Autodesk Inventor part; units mm, degrees
ref_plane "YZ Plane" through (0, 0, 0) normal (1, 0, 0) x (0, 1, 0)
ref_plane "XZ Plane" through (0, 0, 0) normal (0, 1, 0) x (-1, 0, 0)
ref_plane "XY Plane" through (0, 0, 0) normal (0, 0, 1) x (1, 0, 0)
sketch "Sketch1" plane through (0, 0, 0) normal (0, 1, 0) x (-1, 0, 0)
  circle A0 centre (0, 0) radius 20
  circle A1 centre (20, 0) radius 2
  circle A2 centre (10, 17.3205) radius 2
  circle A3 centre (-10, 17.3205) radius 2
  circle A4 centre (-20, 0) radius 2
  circle A5 centre (-10, -17.3205) radius 2
  circle A6 centre (10, -17.3205) radius 2
  circle A7 centre (0, 0) radius 24
  dimension "d16" = 40
  dimension "d17" = 4
  dimension "d20" = 360
  dimension "d22" = 48
extrude "Extrusion1" add sketch "Sketch1" against normal blind 5 contours A0 A1 | A0 A1 | A1 A0 A6 A5 A4 A3 A2 | A2 A0 | A0 A2 | A6 A0 | A0 A6 | A3 A0 | A0 A3 | A5 A0 | A0 A5 | A4 A0 | A0 A4 | A7
sketch "Sketch2" plane through (0, -5, 0) normal (0, -1, 0) x (1, 0, 0)
  circle A0 centre (0, 0) radius 5
  dimension "d13" = 10
extrude "Extrusion3" add sketch "Sketch2" along normal blind 40
extrude "Extrusion4" add sketch "Sketch1" along normal blind 15 contours A0 A1 | A0 A1 | A2 A0 | A0 A2 | A6 A0 | A0 A6 | A3 A0 | A0 A3 | A5 A0 | A0 A5 | A4 A0 | A0 A4
properties part number "Output_shaft"
Input: part model. Units: mm. Frame: model coordinates. A direction names the side the tool comes from. Coordinates: 2 decimals unless noted, no trailing zeros. Loops run counter-clockwise (first coordinate to the right, second up) from the corner with the lowest first, then second, coordinate; pieces in that order, holes last. Notation, with made-up numbers: M -27.5,-36 L -9.5,-36 A20 ccw -9.5,3 Z; hole C 13.5,-27.75 d8. An arc over 180 degrees is marked long. Answer in a Markdown table with one row per item.
1. Section C-C, the plane z = 0. Output: boundary loops of the cut face in (x, y).
Response:
| item | result |
|---|---|
| outline | M -24,-5 L -5,-5 L -5,-45 L 5,-45 L 5,-5 L 24,-5 L 24,0 L 22,0 L 22,15 L 18,15 L 18,0 L -18,0 L -18,15 L -22,15 L -22,0 L -24,0 Z |
2. Reachability of faces 1 (the cylindrical face through (-18.4, 7.4, 1.2)), 2 (the flat face through (0, -5, 6)), 3 (the flat face through (-20, 15, 0)) from +Z, -Z, +X, -X, +Y, -Y: full face, straight path, thin tool, end or side. Return the list, or none.
Response:
| item | result |
|---|---|
| face 1 | +Y |
| face 2 | -Y |
| face 3 | +Z, -Z, +X, -X, +Y |
3. Section A-A, the plane x = 0. Output: boundary loops of the cut face in (y, z).
Response:
| item | result |
|---|---|
| outline | M -45,-5 L -5,-5 L -5,-24 L 0,-24 L 0,24 L -5,24 L -5,5 L -45,5 Z |
4. Section D-D, the plane y = -10.5. Output: boundary loops of the cut face in (x, z), then the cut area to 3 significant figures.
Response:
| item | result |
|---|---|
| outline | C 0,0 d10 |
| area | 78.5 mm2 |
5. Section B-B, the plane y = 2.5. Output: boundary loops of the cut face in (x, z), then the cut area to 3 significant figures.
Response:
| item | result |
|---|---|
| outline | C -20,0 d4; C -10,-17.32 d4; C -10,17.32 d4; C 10,-17.32 d4; C 10,17.32 d4; C 20,0 d4 |
| area | 75.4 mm2 |
6. Draft query along Z for faces 4 (the flat face through (10, 15, 17)), 5 (the cylindrical face through (10.434, 7.395, -15.368)), 6 (the cylindrical face through (-1.08, -24.72, 4.88)). Return one class per face: pulls with the +Z half, pulls with the -Z half, needs draft (parallel to the pull), parting line crosses it, or undercut.
Response:
| item | result |
|---|---|
| face 4 | needs draft |
| face 5 | undercut |
| face 6 | parting line crosses it |
7. Material intervals for line 1 (Y direction, x = -17.5, z = 13); line 2 (Y direction, x = -1, z = 2.5); line 3 (Z direction, x = 1, y = -8.5), sorted ascending.
Response:
| item | result |
|---|---|
| line 1 | y = -5 to 0 |
| line 2 | y = -45 to 0 |
| line 3 | z = -4.9 to 4.9 |
8. First-contact query: pin 1 (3 mm diameter, centred on y = -27, z = -4.5, fed in from +X); pin 2 (2 mm diameter, centred on x = 7.5, z = -3.5, fed in from -Y); pin 3 (10 mm diameter, centred on x = 13.5, y = 1.5, fed in from -Z). Flat tips, straight axial feed; report the tip coordinate or a pass-through.
Response:
| item | result |
|---|---|
| pin 1 | stops at x = 4 |
| pin 2 | stops at y = -5 |
| pin 3 | stops at z = -22.36 |
